```python
from build123d import *
from OCP.BRepFilletAPI import BRepFilletAPI_MakeChamfer

# Parameters (mm, degrees)
SKETCH_2_W            = 20.5
SKETCH_2_H            = 12
EXTRUDE_1_DEPTH       = 50
SKETCH_3_W            = 24
SKETCH_3_H            = 5
CUT_EXTRUDE_1_DEPTH   = 53.431502935
SKETCH_5_W            = 13.122567423
SKETCH_5_H            = 12.5
CUT_EXTRUDE_2_DEPTH   = 53.431502935
SKETCH_7_R            = 0.75
CUT_EXTRUDE_3_DEPTH   = 40.812843405
SKETCH_10_W           = 19.106520138
SKETCH_10_H           = 8.700699496
CUT_EXTRUDE_3_2_DEPTH = 53.431502935
SKETCH_11_R           = 1.5
CUT_EXTRUDE_6_DEPTH   = 54.150729064
SKETCH_9_R            = 1.5
CUT_EXTRUDE_5_DEPTH   = 55.371407927
SKETCH_12_R           = 0.75
CUT_EXTRUDE_4_DEPTH   = 12
CUT_EXTRUDE_7_DEPTH   = 55.371407927
CHAMFER_5_SIZE        = 2
CHAMFER_6_SIZE        = 2
CHAMFER_6_SIZE2       = 1.867573994
CHAMFER_6_SIZE2_2     = 2.1420728
SKETCH_14_R           = 0.75
CUT_EXTRUDE_5_2_DEPTH = 6
CUT_EXTRUDE_8_DEPTH   = 10
SKETCH_16_R           = 0.75
CUT_EXTRUDE_9_DEPTH   = 5


with BuildPart() as part:
    # Эскиз2 → Вытянуть1 (new body)
    with BuildSketch(Plane(origin=(0, 0, 0), x_dir=(0, 0, -1), z_dir=(1, 0, 0))):
        Rectangle(SKETCH_2_W, SKETCH_2_H)
    extrude(amount=EXTRUDE_1_DEPTH)

    # Эскиз3 → Вырез-Вытянуть1 (cut, through all)
    with BuildSketch(Plane(origin=(0, 6, 0), x_dir=(1, 0, 0), z_dir=(0, 1, 0))):
        Rectangle(SKETCH_3_W, SKETCH_3_H)
    extrude(amount=-CUT_EXTRUDE_1_DEPTH, mode=Mode.SUBTRACT)

    # Эскиз5 → Вырез-Вытянуть2 (cut, through all)
    with BuildSketch(Plane(origin=(0, 6, 0), x_dir=(1, 0, 0), z_dir=(0, 1, 0))):
        with Locations((44.561283712, 0)):
            Rectangle(SKETCH_5_W, SKETCH_5_H)
    extrude(amount=-CUT_EXTRUDE_2_DEPTH, mode=Mode.SUBTRACT)

    # Эскиз7 → Cut-Extrude 3 (cut, through all)
    with BuildSketch(Plane(origin=(38, 0, 0), x_dir=(0, 0, -1), z_dir=(1, 0, 0))):
        with Locations((0, 3)):
            Circle(SKETCH_7_R)
    extrude(amount=-CUT_EXTRUDE_3_DEPTH, mode=Mode.SUBTRACT)

    # Эскиз10 → Cut-Extrude 3 2 (cut, through all)
    with BuildSketch(Plane(origin=(0, 6, 0), x_dir=(1, 0, 0), z_dir=(0, 1, 0))):
        with Locations((3.446739931, 11.100349748)):
            Rectangle(SKETCH_10_W, SKETCH_10_H)
        with Locations((3.446739931, -11.100349748)):
            Rectangle(SKETCH_10_W, SKETCH_10_H)
    extrude(amount=-CUT_EXTRUDE_3_2_DEPTH, mode=Mode.SUBTRACT)

    # Эскиз11 → Вытянуть6 (cut, through all)
    with BuildSketch(Plane.XY.offset(6.75)):
        with Locations((5, -1)):
            Circle(SKETCH_11_R)
    extrude(amount=-CUT_EXTRUDE_6_DEPTH, mode=Mode.SUBTRACT)

    # Эскиз9 → Cut-Extrude 5 (cut, through all)
    with BuildSketch(Plane.XY.offset(10.25)):
        with Locations((45.5, -1.5)):
            Circle(SKETCH_9_R)
    extrude(amount=-CUT_EXTRUDE_5_DEPTH, mode=Mode.SUBTRACT)

    # Эскиз12 → Вырез-Вытянуть4 (cut)
    with BuildSketch(Plane.ZY.offset(-12)):
        with Locations((-1.791386219, -3.407348241)):
            Circle(SKETCH_12_R)
    extrude(amount=-CUT_EXTRUDE_4_DEPTH, mode=Mode.SUBTRACT)

    # Эскиз13 → Вытянуть7 (cut, through all)
    with BuildSketch(Plane.XY.offset(10.25)):
        Polygon((13, 6), (0, 6), (0, 2), align=None)
        Polygon((50, 6), (50, 1), (38, 6), align=None)
    extrude(amount=-CUT_EXTRUDE_7_DEPTH, mode=Mode.SUBTRACT)

    # Фаска5
    chamfer_5_edges = [part.edges().sort_by_distance(p)[0] for p in [
        (50, -6, 8.25),
        (0, -6, -4.625),
        (50, -6, -8.25),
        (0, -6, 4.625),
    ]]
    chamfer(chamfer_5_edges, length=CHAMFER_5_SIZE)

    # Фаска6: one chamfer whose edges measure the first distance from different faces: ONE call of the kernel's chamfer builder (chamfer() names one face for all edges)
    chamfer_6_edges_1 = [part.edges().sort_by_distance(p)[0] for p in [
        (0, 2, 4.625),
    ]]
    chamfer_6_side_1 = [part.faces().sort_by_distance(p)[0] for p in [
        (0, -1, 4.625),
    ]]
    chamfer_6_edges_2 = [part.edges().sort_by_distance(p)[0] for p in [
        (0, 2, -4.625),
    ]]
    chamfer_6_side_2 = [part.faces().sort_by_distance(p)[0] for p in [
        (0, -1, -4.625),
    ]]
    chamfer_6_edges_3 = [part.edges().sort_by_distance(p)[0] for p in [
        (50, 1, 8.25),
    ]]
    chamfer_6_side_3 = [part.faces().sort_by_distance(p)[0] for p in [
        (44, 3.5, 8.25),
    ]]
    chamfer_6_edges_4 = [part.edges().sort_by_distance(p)[0] for p in [
        (50, 1, -8.25),
    ]]
    chamfer_6_side_4 = [part.faces().sort_by_distance(p)[0] for p in [
        (44, 3.5, -8.25),
    ]]
    chamfer_6 = BRepFilletAPI_MakeChamfer(part.part.solid().wrapped)
    for e in chamfer_6_edges_1:
        chamfer_6.Add(CHAMFER_6_SIZE, CHAMFER_6_SIZE2, e.wrapped, chamfer_6_side_1[0].wrapped)  # the first distance lies on this face
    for e in chamfer_6_edges_2:
        chamfer_6.Add(CHAMFER_6_SIZE, CHAMFER_6_SIZE2, e.wrapped, chamfer_6_side_2[0].wrapped)  # the first distance lies on this face
    for e in chamfer_6_edges_3:
        chamfer_6.Add(CHAMFER_6_SIZE, CHAMFER_6_SIZE2_2, e.wrapped, chamfer_6_side_3[0].wrapped)  # the first distance lies on this face
    for e in chamfer_6_edges_4:
        chamfer_6.Add(CHAMFER_6_SIZE, CHAMFER_6_SIZE2_2, e.wrapped, chamfer_6_side_4[0].wrapped)  # the first distance lies on this face
    add(Compound.cast(chamfer_6.Shape()), mode=Mode.REPLACE)

    # Эскиз14 → Cut-Extrude 5 2 (cut)
    with BuildSketch(Plane(origin=(38, 0, 0), x_dir=(0, 0, -1), z_dir=(1, 0, 0))):
        with Locations((-2, -3.75)):
            Circle(SKETCH_14_R)
    extrude(amount=-CUT_EXTRUDE_5_2_DEPTH, mode=Mode.SUBTRACT)

    # Эскиз15 → Вытянуть8 (cut)
    with BuildSketch(Plane.XZ.offset(6)):
        with BuildLine():
            Line((18, 6.25), (32, 6.25))
            ThreePointArc((32, 6.25), (34.121320344, 5.371320344), (35, 3.25))
            Line((35, 3.25), (35, -3.25))
            ThreePointArc((35, -3.25), (34.121320344, -5.371320344), (32, -6.25))
            Line((32, -6.25), (18, -6.25))
            ThreePointArc((18, -6.25), (15.878679656, -5.371320344), (15, -3.25))
            Line((15, -3.25), (15, 3.25))
            ThreePointArc((15, 3.25), (15.878679656, 5.371320344), (18, 6.25))
        make_face()
    extrude(amount=-CUT_EXTRUDE_8_DEPTH, mode=Mode.SUBTRACT)

    # Эскиз16 → Вытянуть9 (cut)
    with BuildSketch(Plane.ZY.offset(-12)):
        with Locations((1.748401574, 3.000943563)):
            Circle(SKETCH_16_R)
    extrude(amount=-CUT_EXTRUDE_9_DEPTH, mode=Mode.SUBTRACT)


solid = part.part
```
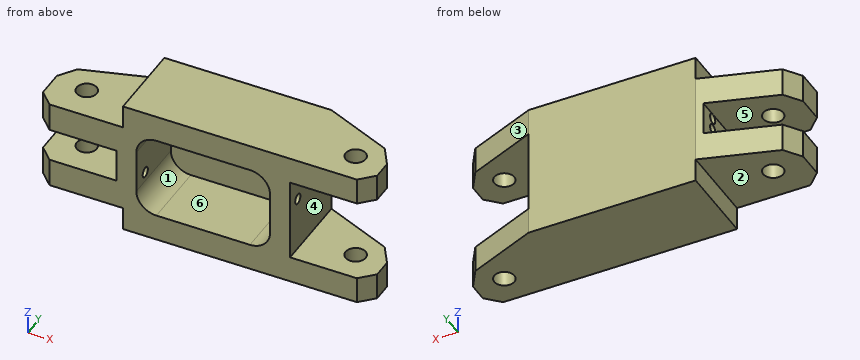
Check sheet for the modelled part. Datum: model origin and axes. Units: mm. Face numbers are marked on the shaded views. A direction names the side the tool comes from. Give positions to 0.01 mm unless a question says otherwise; leave off trailing zeros. Write each loop counter-clockwise with the first axis right and the second up, starting at its lowest first coordinate (ties: lowest second). Pieces come first, ordered by that corner, then holes. Notation, with made-up numbers: (-14, 16.5) -> (32, 16.5) arc R19 ccw to (32, 41.5) -> close; hole circle Ø9 at (37, 57). An arc over 180 degrees is marked (long way). Use CSV: the item, a comma, the result in double quotes. Start each with the question number.
Q1. Tool access check on the marked faces 4, 5 and 6. Record the directions out of +Z, -Z, +X, -X, +Y, -Y that give a thin tool (end or side, any length) a straight path to the whole face; none if there is none.
Q2. Cross-section at C-C on x = 26. Enter the section's corners in (y, z), and give its area (3 significant figures).
Q3. Release check for a two-part mould opening along Z. For the marked faces 1, 2 and 3 record: +Z half, -Z half, draft (parallel to the pull), parting line (faces both ways), or undercut.
Q4. Cross-section at A-A on z = 0. Enter the section's corners in (x, y).
Q5. Cross-section at B-B on y = 5. Enter the section's corners in (x, z), and give its area (3 significant figures).
Q6. Depth check by flat-ended pin: P1, Ø1.2, axis at y = -3.41, z = -1.79, coming from the +X side; P2, Ø3.5, axis at x = 5, y = -1, coming from the +Z side; P3, Ø2.5, axis at x = 45.5, y = -1.5, coming from the +Z side; P4, Ø3.5, axis at x = 45.5, y = -1.5, coming from the +Z side. Enter the tip coordinate at first touch or a pass-through.
Q7. Scan lines: line 1 along Y through (x, z) = (37.05, 2); line 2 along Z through (x, y) = (47.5, -5.25); line 3 along Z through (x, y) = (9, -2.25). Record each from-to range of solid material in increasing order.
Q8. Cross-section at D-D on z = 8.5. Enter the section's corners in (x, y), and give its area (3 significant figures).
Working result:
1,face 4,"+X, +Y, -Y"
1,face 5,"-X, +Y, -Y"
1,face 6,"-Y"
2,outline,"(-6, -10.25) -> (6, -10.25) -> (6, 10.25) -> (-6, 10.25) -> (-6, 6.25) -> (4, 6.25) -> (4, -6.25) -> (-6, -6.25) -> close"
2,area,"121 mm^2"
3,face 1,"undercut"
3,face 2,"-Z half"
3,face 3,"draft"
4,outline,"(12, -6) -> (15, -6) -> (15, 2.25) -> (12, 2.25) -> close; (12, 3.75) -> (15, 3.75) -> (15, 4) -> (35, 4) -> (35, 3.75) -> (38, 3.75) -> (38, 6) -> (13, 6) -> (12, 5.69) -> close; (35, -6) -> (38, -6) -> (38, 2.25) -> (35, 2.25) -> close"
5,outline,"(9.75, -6.75) -> (13, -6.75) -> (13, -10.25) -> (40.4, -10.25) -> (40.4, -6.25) -> (38, -6.25) -> (38, 6.25) -> (40.4, 6.25) -> (40.4, 10.25) -> (13, 10.25) -> (13, 6.75) -> (9.75, 6.75) -> (9.75, 2.5) -> (12, 2.5) -> (12, -2.5) -> (9.75, -2.5) -> close"
5,area,"564 mm^2"
6,P1,"stops at x = 38"
6,P2,"stops at z = 6.75"
6,P3,"passes through"
6,P4,"stops at z = 10.25"
7,line 1,"y = -6 to -4.5, -3 to 6"
7,line 2,"z = -10.25 to -6.25, 6.25 to 10.25"
7,line 3,"z = -6.75 to -2.5, 2.5 to 6.75"
8,outline,"(13, -6) -> (48, -6) -> (50, -4) -> (50, -1.14) -> (48.15, 1.77) -> (38, 6) -> (13, 6) -> close; hole circle Ø3 at (45.5, -1.5)"
8,area,"403 mm^2"
